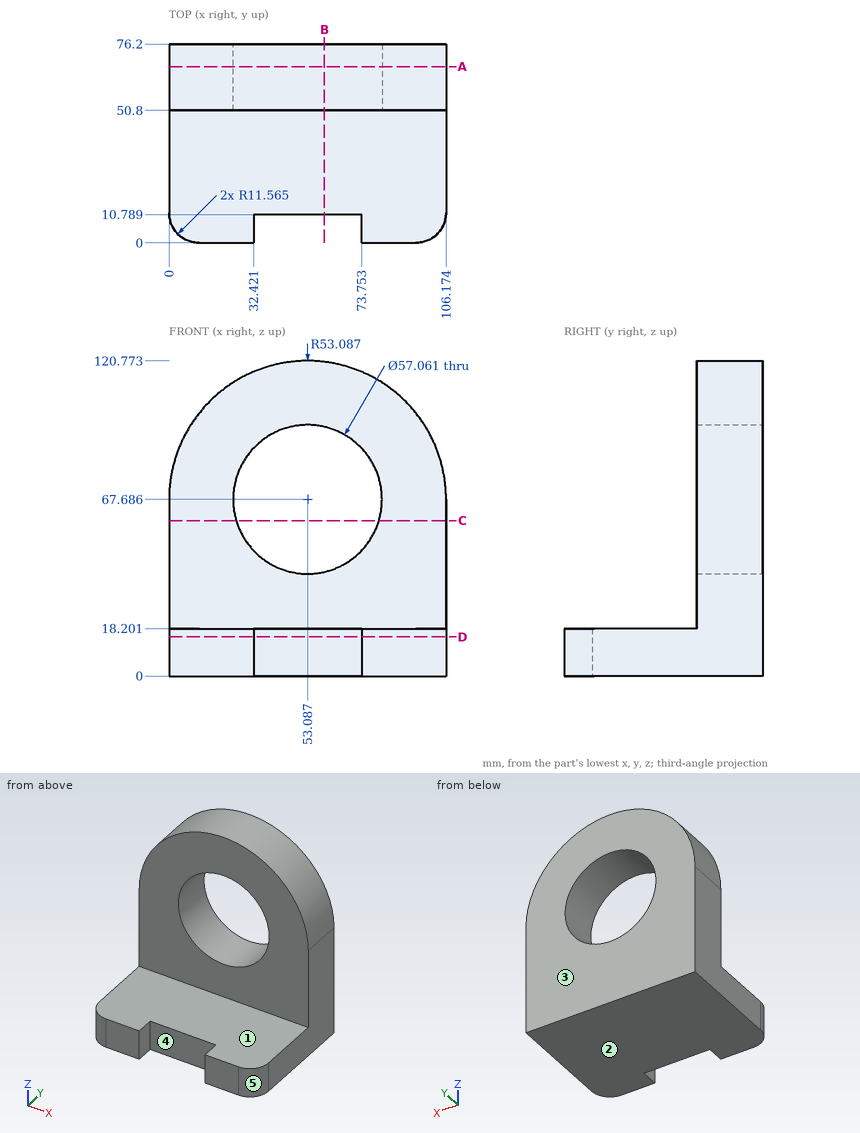
Could you check a few things on this drawing? It's one solid part, dimensions in mm from its lowest x, y, z. A direction names the side the tool comes from. Coordinates: 2 decimals unless noted, no trailing zeros. Write each loop counter-clockwise with the first axis right and the second up, starting at its lowest first coordinate (ties: lowest second). Pieces come first, ordered by that corner, then holes.
1) If we section it at A-A (y = 67.5): List the corners of the cut face in (x, z) for me (1 decimal).
Filled in:
outline: (0, 0) - (106.2, 0) - (106.2, 67.7) arc R53.1 ccw to (0, 67.7) - close; hole circle Ø57.1 at (53.1, 67.7)
2) If I drill on line 1 (Y direction, x = 8, z = 21); line 2 (Z direction, x = 32, y = 54.5) (1 decimal); line 3 (Z direction, x = 77.5, y = 48), over which ranges is the centre line in solid material (lowest first)?
Filled in:
line 1: y = 50.8 to 76.2
line 2: z = 0 to 48.5, 86.9 to 116.4
line 3: z = 0 to 18.2
3) Thinking about a two-plate mould opening in X: for the marked faces 3, 4 and 5, which applies, +X half, -X half, draft (parallel to the pull), parting line (faces both ways), or undercut?
Filled in:
face 3: draft
face 4: undercut
face 5: +X half
4) If we section it at D-D (z = 15): List the corners of the cut face in (x, y) for me (1 decimal).
Filled in:
outline: (0, 11.6) arc R11.6 ccw to (11.6, 0) - (32.4, 0) - (32.4, 10.8) - (73.8, 10.8) - (73.8, 0) - (94.6, 0) arc R11.6 ccw to (106.2, 11.6) - (106.2, 76.2) - (0, 76.2) - close
5) If we section it at B-B (x = 59.5): List the corners of the cut face in (y, z) for me (1 decimal).
Filled in:
outline: (10.8, 0) - (76.2, 0) - (76.2, 39.9) - (50.8, 39.9) - (50.8, 18.2) - (10.8, 18.2) - close; (50.8, 95.5) - (76.2, 95.5) - (76.2, 120.4) - (50.8, 120.4) - close
6) If we section it at C-C (z = 59.5): List the corners of the cut face in (x, y) for me (1 decimal).
Filled in:
outline: (0, 50.8) - (25.8, 50.8) - (25.8, 76.2) - (0, 76.2) - close; (80.4, 50.8) - (106.2, 50.8) - (106.2, 76.2) - (80.4, 76.2) - close
7) Which directions (+Z, -Z, +X, -X, +Y, -Y) give clear straight access to the entire face, cutting with the end or side of a thin tool? Please do the marked faces 1 and 2.
Filled in:
face 1: +Z, +X, -X, -Y
face 2: -Z, +X, -X, +Y, -Y
8) I'm going to push flat-ended pins straight in: pin 1 (1 mm diameter, centred on y = 55, z = 75.5, fed in from -X); pin 2 (5 mm diameter, centred on y = 50, z = 106, fed in from -X); pin 3 (8.5 mm diameter, centred on y = 3.5, z = 11.5, fed in from -X). Where does each tip first touch, or does it pass through?
Filled in:
pin 1: stops at x = 0.51
pin 2: stops at x = 14.02
pin 3: stops at x = 0.65
